Autodesk Inventor part; units mm, degrees
ref_plane "YZ Plane" through (0, 0, 0) normal (1, 0, 0) x (0, 1, 0)
ref_plane "XZ Plane" through (0, 0, 0) normal (0, 1, 0) x (-1, 0, 0)
ref_plane "XY Plane" through (0, 0, 0) normal (0, 0, 1) x (1, 0, 0)
ref_plane "Work Plane1" through (0, 0, 0) normal (0, 0, 1) x (1, 0, 0)
sketch "Sketch1" plane through (0, 0, 0) normal (0, 0, 1) x (1, 0, 0)
  circle A0 centre (0, 14.168) radius 14
  circle A1 centre (8, 14.168) radius 2.45
  circle A2 centre (-8, 14.168) radius 2.45
  circle A3 centre (0, 14.168) radius 14
  circle A4 centre (0, 6.168) radius 2.45
  circle A5 centre (0, 22.168) radius 2.45
  point P0 (0, 0)
  dimension "d0" = 4.9
  dimension "d1" = 4.9
  dimension "d2" = 8
  dimension "d3" = 8
  dimension "d9" = 4.9
  dimension "d10" = 4.9
  dimension "d11" = 8
  dimension "d12" = 8
extrude "Extrusion1" add sketch "Sketch1" along normal blind 20
sketch "Sketch2" plane through (0, 14.168, 20) normal (0, 0, 1) x (1, 0, 0)
  circle A0 centre (-8, 0) radius 2.45
  circle A1 centre (8, 0) radius 2.45
  circle A2 centre (0, 0) radius 14
  circle A3 centre (0, -45.639) radius 6.15 construction
  circle A4 centre (0, -45.639) radius 2.5
  line L0 (6.0583, -46.6969) -> (13.7914, -2.408)
  line L1 (-6.0583, -46.6969) -> (-13.7914, -2.408)
  circle A5 centre (0, 0) radius 14
  arc A6 (-6.0583, -46.6969) -> (6.0583, -46.6969) centre (0, -45.639) ccw
  point P0 (0, -14.168)
  dimension "d6" = 5
extrude "Extrusion2" add sketch "Sketch2" along normal blind 5 contours A0 | A1 | A2 | A2 L0 A6 L1
properties part number "20_Cube_Insert_Z-focus_Single_LED_arm"
The model under review builds one solid part; all positions refer to its coordinate system, in mm. A direction names the side the tool comes from. Round coordinates to 2 decimals unless told otherwise and drop trailing zeros. Write each loop counter-clockwise with the first axis right and the second up, starting at its lowest first coordinate (ties: lowest second). Pieces come first, ordered by that corner, then holes. Notation, with made-up numbers: (1, -12) - (59, -12) arc R21 ccw to (59, 21) - close; hole circle Ø4 at (-27, -37.75). An arc over 180 degrees is marked (long way). One line per question, with ' | ' between items.
Item 1: For faces 1 (the face through (-8.32, 11.74, 9.86)), 2 (the face through (-0.33, -33.95, 22.46)), list the 3-axis set-ups (+Z, -Z, +X, -X, +Y, -Y) from which the entire face can be reached by the end or side of a thin tool; tool diameter is ignored.
Resolved:
face 1: -Z | face 2: +Z, -Z
Item 2: The part is to be moulded in two halves that separate along X. For faces 3 (the face through (0, 22, 20)), 4 (the face through (0.12, -37.62, 22.46)), 5 (the face through (0, 14, 0)), 6 (the face through (-9.87, -10.69, 22.46)), say which applies: pulls with the +X half, pulls with the -X half, needs draft (parallel to the pull), parting line crosses it, or undercut.
Resolved:
face 3: undercut | face 4: parting line crosses it | face 5: needs draft | face 6: pulls with the -X half
Item 3: To check wall thickness, follow probe 1 along Y at (x, z) = (0, 5.75); probe 2 along Y at (x, z) = (2, 19.25); probe 3 along Y at (x, z) = (0, 23.1). State the ranges of each line that lie inside material, in increasing order.
Resolved:
probe 1: y = 0.17 to 3.72, 8.62 to 19.72, 24.62 to 28.17 | probe 2: y = 0.31 to 4.75, 7.58 to 20.75, 23.58 to 28.02 | probe 3: y = -37.62 to -33.97, -28.97 to 28.17
Item 4: Add section D-D, the plane y = -7. Give the boundary of the cut face in (x, z), then the cut area to 3 significant figures.
Resolved:
outline: (-10.52, 20) - (10.52, 20) - (10.52, 25) - (-10.52, 25) - close | area: 105 mm2
Item 5: Add section A-A, the plane z = 21.5. Give the boundary of the cut face in (x, y), then the cut area to 3 significant figures.
Resolved:
outline: (-13.79, 11.76) - (-6.06, -32.53) arc R6.15 ccw to (6.06, -32.53) - (13.79, 11.76) arc R14 ccw (long way) to start; hole circle Ø5 at (0, -31.47) | area: 1,280 mm2
Item 6: For P1, Ø12, axis at x = -3.5, z = 20, coming from the -Y side; P2, Ø4.5, axis at x = 8, y = 14.168, coming from the -Z side; P3, Ø10, axis at y = -1.5, z = 6, coming from the +X side; P4, Ø3, axis at x = 0, y = -31.471, coming from the +Z side, all flat-tipped, find the tip position at first contact; note any pin that passes through.
Resolved:
P1: stops at y = -37.62 | P2: stops at z = 20 | P3: stops at x = 9.07 | P4: passes through
Item 7: Add section C-C, the plane z = 5.75. Give the boundary of the cut face in (x, y), then the cut area to 3 significant figures.
Resolved:
outline: circle Ø28 at (0, 14.17); hole circle Ø4.9 at (-8, 14.17); hole circle Ø4.9 at (0, 6.17); hole circle Ø4.9 at (0, 22.17); hole circle Ø4.9 at (8, 14.17) | area: 540 mm2
